Part model, mm, in its own coordinate system. A direction names the side the tool comes from. Round coordinates to 2 decimals unless told otherwise and drop trailing zeros. Loops run counter-clockwise (first coordinate to the right, second up) from the corner with the lowest first, then second, coordinate; pieces in that order, holes last.
(1) Cut at D-D on z = 10.75. List the corners of the cut face in (x, y).
(2) Cut at B-B on z = -1.25. List the corners of the cut face in (x, y).
(3) Tool access for faces 4 (the face through (30.1, 0.1, -7.4)), 5 (the face through (-12.302, -2.069, 2.994)): list every direction of +Z, -Z, +X, -X, +Y, -Y with a clear straight run to the whole face (end or side of a thin tool).
(4) Flat gauge pins, fed straight in: pin 1 (4 mm diameter, centred on x = -15, y = 0, fed in from +Z); pin 2 (9 mm diameter, centred on x = 25, z = 2.5, fed in from +Y); pin 3 (10 mm diameter, centred on x = -26.5, z = -4.5, fed in from +Y). Where does each tip first touch, or does it go through?
(5) Probe probe 1 along Z at (x, y) = (25, -1); probe 2 along Y at (x, z) = (-15, -4.5); probe 3 along X at (y, z) = (-5.25, 1.75). List the from-to ranges inside material, lowest first.
(6) Cut at C-C on z = 4. List the corners of the cut face in (x, y).
(7) Mould opens along Y. For faces 1 (the face through (20.005, -0.112, 2.72)), 2 (the face through (15.56, 0.18, -7.94)), 3 (the face through (0, -8, 0)) say: +Y half, -Y half, draft (parallel to the pull), parting line (faces both ways), or undercut.
(8) Cut at A-A on x = -25. List the corners of the cut face in (y, z), then the cut area to 3 significant figures.
from build123d import *

# Parameters (mm, degrees)
F0_W     = 70
F0_H     = 25
F1_DEPTH = 8
F2_SIZE  = 5
F3_SIZE  = 10
F4_R     = 5
F5_DEPTH = 16
F7_D     = 6.8
F7_DEPTH = 18.75
F7_TIP   = 2.0429261047


with BuildPart() as f1:
    # F0 (on Front) → F1 (new body, symmetric)
    with BuildSketch(Plane.XZ):
        Rectangle(F0_W, F0_H)
    extrude(amount=F1_DEPTH, both=True)

    # F2
    f2_edges = [f1.edges().sort_by_distance(p)[0] for p in [
        (-35, 0, -12.5),
    ]]
    chamfer(f2_edges, length=F2_SIZE)

    # F3
    f3_edges = [f1.edges().sort_by_distance(p)[0] for p in [
        (35, 0, -12.5),
    ]]
    chamfer(f3_edges, length=F3_SIZE)

    # F4 (on face) → F5 (cut)
    with BuildSketch(Plane.XZ.offset(8)):
        with Locations((-25, -2.5)):
            Circle(F4_R)
        with Locations((25, 2.5)):
            Circle(F4_R)
    extrude(amount=-F5_DEPTH, mode=Mode.SUBTRACT)

    # F7
    with Locations(Plane.XY.offset(12.5)):
        with Locations((-15, 0), (15, 0)):
            Hole(F7_D / 2, depth=F7_DEPTH)
            with Locations((0, 0, -(F7_DEPTH + F7_TIP / 2))):  # 118° drill point
                Cone(0, F7_D / 2, F7_TIP, mode=Mode.SUBTRACT)


solid = f1.part
Final values:
1. outline: (-35, -8) - (35, -8) - (35, 8) - (-35, 8) - close; hole circle Ø6.8 at (-15, 0); hole circle Ø6.8 at (15, 0)
2. outline: (-35, -8) - (-29.84, -8) - (-29.84, 8) - (-35, 8) - close; (-20.16, -8) - (21.69, -8) - (21.69, 8) - (-20.16, 8) - close; (28.31, -8) - (35, -8) - (35, 8) - (28.31, 8) - close; hole circle Ø6.8 at (-15, 0); hole circle Ø6.8 at (15, 0)
3. face 4: -Z, +X, +Y, -Y
3. face 5: +Z
4. pin 1: stops at z = -7.09
4. pin 2: passes through
4. pin 3: stops at y = 8
5. probe 1: z = -12.5 to -2.5, 7.5 to 12.5
5. probe 2: y = -8 to -3.4, 3.4 to 8
5. probe 3: x = -35 to -27.63, -22.37 to 20.06, 29.94 to 35
6. outline: (-35, -8) - (20.23, -8) - (20.23, 8) - (-35, 8) - close; (29.77, -8) - (35, -8) - (35, 8) - (29.77, 8) - close; hole circle Ø6.8 at (-15, 0); hole circle Ø6.8 at (15, 0)
7. face 1: draft
7. face 2: undercut
7. face 3: -Y half
8. outline: (-8, -12.5) - (8, -12.5) - (8, -7.5) - (-8, -7.5) - close; (-8, 2.5) - (8, 2.5) - (8, 12.5) - (-8, 12.5) - close
8. area: 240 mm2
